```python
from build123d import *

# Parameters (mm, degrees)
SKETCH1_R           = 2.54
BOSS_EXTRUDE1_DEPTH = 5.08
SKETCH2_R           = 22.825529453
BOSS_EXTRUDE2_DEPTH = 33.02
SKETCH3_R           = 2.54
CUT_EXTRUDE1_DEPTH  = 39.1
BOSS_EXTRUDE3_DEPTH = 5.08
SKETCH5_R           = 2.54
CUT_EXTRUDE2_DEPTH  = 39.1


with BuildPart() as part:
    # Sketch1 → Boss-Extrude1 (new body)
    with BuildSketch(Plane.XY):
        with BuildLine():
            Line((-16.891, -131.282672274), (16.891, -131.282672274))
            ThreePointArc((16.891, -131.282672274), (19.601252021, -114.911473805), (27.442816508, -100.287128633))
            ThreePointArc((27.442816508, -100.287128633), (30.785280347, -96.37410804), (34.5064888, -92.819336271))
            ThreePointArc((34.5064888, -92.819336271), (0, 0), (-34.5064888, -92.819336271))
            ThreePointArc((-34.5064888, -92.819336271), (-30.785280347, -96.37410804), (-27.442816508, -100.287128633))
            ThreePointArc((-27.442816508, -100.287128633), (-19.601252021, -114.911473805), (-16.891, -131.282672274))
        make_face()
        with Locations((-10.756405179, -114.872047193)):
            Circle(SKETCH1_R, mode=Mode.SUBTRACT)
        with Locations((10.756405179, -114.872047193)):
            Circle(SKETCH1_R, mode=Mode.SUBTRACT)
    extrude(amount=BOSS_EXTRUDE1_DEPTH)

    # Sketch2 → Boss-Extrude2 (add)
    with BuildSketch(Plane(origin=(0, 0, 0), x_dir=(-1, 0, 0), z_dir=(0, 0, -1))):
        with Locations((0, -52.823729134)):
            Circle(SKETCH2_R)
    extrude(amount=BOSS_EXTRUDE2_DEPTH)

    # Sketch3 → Cut-Extrude1 (cut, through all)
    with BuildSketch(Plane(origin=(0, 0, -33.02), x_dir=(-1, 0, 0), z_dir=(0, 0, -1))):
        with Locations((0, -52.823729134)):
            Circle(SKETCH3_R)
    extrude(amount=-CUT_EXTRUDE1_DEPTH, mode=Mode.SUBTRACT)

    # Sketch4 → Boss-Extrude3 (add)
    with BuildSketch(Plane.XY.offset(5.08)):
        with BuildLine():
            ThreePointArc((45.161811227, -80.223677424), (52.45816234, -46.619894549), (37.524583334, -15.645079276))
            add(Edge.make_bspline(
                [(37.524583334, -15.645079276), (41.569282444, -19.727412804), (51.389708048, -24.415182371), (63.297197231, -26.895437115), (68.900180003, -24.949874899)],
                knots=[0, 0, 0, 0, 0.479929933, 1, 1, 1, 1], degree=3))
            ThreePointArc((68.900180003, -24.949874899), (98.354072, -43.866775297), (72.9914133, -67.993864183))
            add(Edge.make_bspline(
                [(45.161811227, -80.223677424), (47.574313167, -76.247284621), (55.033388576, -68.640688731), (65.508215076, -66.903538588), (72.9914133, -67.993864183)],
                knots=[0, 0, 0, 0, 0.395495141, 1, 1, 1, 1], degree=3))
        make_face()
    extrude(amount=-BOSS_EXTRUDE3_DEPTH)

    # Sketch5 → Cut-Extrude2 (cut, through all)
    with BuildSketch(Plane.XY.offset(5.08)):
        with Locations((76.2, -45.972469461)):
            Circle(SKETCH5_R)
    extrude(amount=-CUT_EXTRUDE2_DEPTH, mode=Mode.SUBTRACT)


solid = part.part
```
Design review of the part built by this model. Coordinates are the model's own, in mm. A direction names the side the tool comes from. Give positions to 0.01 mm unless a question says otherwise; leave off trailing zeros. Loops run counter-clockwise (first coordinate to the right, second up) from the corner with the lowest first, then second, coordinate; pieces in that order, holes last. Notation, with made-up numbers: M 35.25,-7 L 39.25,-7 A19 ccw 39.25,25 Z; hole C 89,-30 d8. An arc over 180 degrees is marked long. Return JSON: item names as keys, results as strings. Group by question number.
Item 1: We need section D-D (y = -41.5). Give the boundary of the cut face in (x, z).
Item 2: Tool access review of faces 4 (the flat face through (22, -65, 0)), 5 (the cylindrical face through (10.426, -112.354, 2.504)): name each direction out of +Z, -Z, +X, -X, +Y, -Y from which nothing blocks a thin tool from reaching the whole face with its end or side.
Item 3: We need section B-B (x = 0). Give the boundary of the cut face in (y, z), and give its area (3 significant figures).
Item 4: We need section A-A (x = 76.2). Give the boundary of the cut face in (y, z), and give its area (3 significant figures).
Item 5: For probe 1 along Y at (x, z) = (0, -18); probe 2 along Y at (x, z) = (76.2, 2.7); probe 3 along Z at (x, y) = (-6.5, -9.5), list the stretches that pass through material, from the lowest coordinate up.
Item 6: Mouldability with a two-part tool opening along Y and no side actions: class faces 1 (the flat face through (5, -65, 5.08)), 2 (the cylindrical face through (4.948, -75.106, -16.279)), 3 (the cylindrical face through (-11.087, -112.354, 2.504)) as released by +Y, released by -Y, zero draft, split by the parting line, or undercut.
Item 7: We need section C-C (z = -15.5). Give the boundary of the cut face in (x, y).
Item 8: Insertion check: pin 1 Ø4 at (x, y) = (-18.5, -19.5) entering from -Z; pin 2 Ø1.5 at (x, z) = (9.5, -5.5) entering from -Y; pin 3 Ø4 at (x, z) = (-18.5, -28.5) entering from -Y. Each pin has a flat end and moves straight along its axis. Give the tip position at first contact, or say it passes through.
Output:
{
 "1": {"outline": "M -51.6,0 L -19.82,0 L -19.82,-33.02 L 19.82,-33.02 L 19.82,0 L 98,0 L 98,5.08 L -51.6,5.08 Z"},
 "2": {"face 4": "-Z", "face 5": "+Z, -Z"},
 "3": {"outline": "M -131.28,0 L -75.65,0 L -75.65,-33.02 L -55.36,-33.02 L -55.36,5.08 L -131.28,5.08 Z; M -50.28,-33.02 L -30,-33.02 L -30,0 L 0,0 L 0,5.08 L -50.28,5.08 Z", "area": "1,980 mm^2"},
 "4": {"outline": "M -68.23,0 L -48.51,0 L -48.51,5.08 L -68.23,5.08 Z; M -43.43,0 L -23.72,0 L -23.72,5.08 L -43.43,5.08 Z", "area": "200 mm^2"},
 "5": {"probe 1": "y = -75.65 to -55.36, -50.28 to -30", "probe 2": "y = -68.23 to -48.51, -43.43 to -23.72", "probe 3": "z = 0 to 5.08"},
 "6": {"face 1": "zero draft", "face 2": "split by the parting line", "face 3": "undercut"},
 "7": {"outline": "C 0,-52.82 d45.65; hole C 0,-52.82 d5.08"},
 "8": {"pin 1": "stops at z = 0", "pin 2": "stops at y = -73.91", "pin 3": "stops at y = -68.6"}
}
